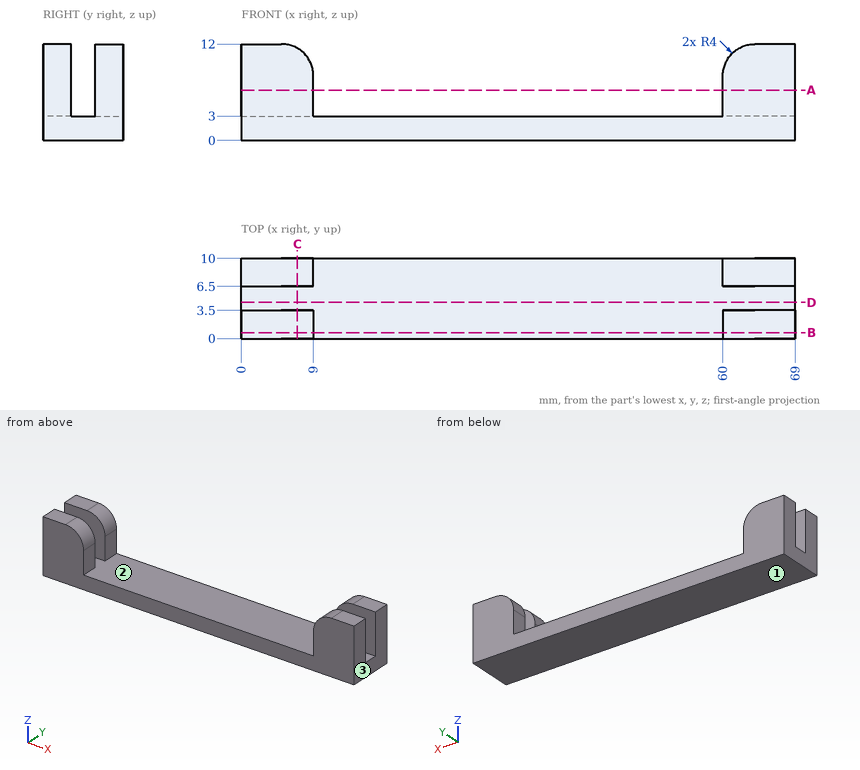
Geometry check sheet. Reference: drawing and pictorial views, mm from the part's lowest x, y, z. Round coordinates to 2 decimals unless told otherwise and drop trailing zeros. Loops run counter-clockwise (first coordinate to the right, second up) from the corner with the lowest first, then second, coordinate; pieces in that order, holes last. Notation, with made-up numbers: M 12,-38.5 L 17,-38.5 A17 cw 17,-5.5 Z; hole C 8.25,55.25 d2. An arc over 180 degrees is marked long. One line per item, written item: value.
(1) Sectioned sample at D-D, the plane y = 4.5. Record the cut outline in (x, z), then the cut area to 3 significant figures.
Computed values:
outline: M 0,0 L 69,0 L 69,3 L 0,3 Z
area: 207 mm^2
(2) Depth check by flat-ended pin: pin 1 Ø3 at (x, y) = (53.5, 4) entering from -Z; pin 2 Ø1.5 at (x, y) = (56, 1) entering from +Z. Enter the tip coordinate at first touch or a pass-through.
Computed values:
pin 1: stops at z = 0
pin 2: stops at z = 3
(3) Thickness scan on line 1 (X direction, y = 8, z = 5); line 2 (Z direction, x = 33, y = 3.25); line 3 (X direction, y = 2, z = 8.75). Record the ranges inside material, lowest first.
Computed values:
line 1: x = 0 to 9, 60 to 69
line 2: z = 0 to 3
line 3: x = 0 to 8.93, 60.07 to 69
(4) Sectioned sample at A-A, the plane z = 6.25. Record the cut outline in (x, y), then the cut area to 3 significant figures.
Computed values:
outline: M 0,0 L 9,0 L 9,3.5 L 0,3.5 Z; M 0,6.5 L 9,6.5 L 9,10 L 0,10 Z; M 60,0 L 69,0 L 69,3.5 L 60,3.5 Z; M 60,6.5 L 69,6.5 L 69,10 L 60,10 Z
area: 126 mm^2
(5) Sectioned sample at B-B, the plane y = 0.75. Record the cut outline in (x, z), then the cut area to 3 significant figures.
Computed values:
outline: M 0,0 L 69,0 L 69,12 L 64,12 A4 ccw 60,8 L 60,3 L 9,3 L 9,8 A4 ccw 5,12 L 0,12 Z
area: 362 mm^2
(6) Sectioned sample at C-C, the plane x = 7. Record the cut outline in (y, z), then the cut area to 3 significant figures.
Computed values:
outline: M 0,0 L 10,0 L 10,11.46 L 6.5,11.46 L 6.5,3 L 3.5,3 L 3.5,11.46 L 0,11.46 Z
area: 89.2 mm^2
(7) Release check for a two-part mould opening along X. For the marked faces 1, 2 and 3 record: +X half, -X half, draft (parallel to the pull), parting line (faces both ways), or undercut.
Computed values:
face 1: draft
face 2: undercut
face 3: +X half
